Here's how the part is built. I have some questions about the finished solid (model axes, mm). A direction names the side the tool comes from. Give positions to 0.01 mm unless a question says otherwise; leave off trailing zeros. Write each loop counter-clockwise with the first axis right and the second up, starting at its lowest first coordinate (ties: lowest second). Pieces come first, ordered by that corner, then holes. Notation, with made-up numbers: (-26, 63) -> (-20, 63) arc R27 cw to (-20, 96) -> close; hole circle Ø10 at (18.25, 16.25). An arc over 180 degrees is marked (long way). Use CSV: the item, a comma, the result in double quotes. Start each with the question number.
(1) Suppose I cut it at C-C on y = 40. List the corners of the cut face in (x, z) for me, plus the area to 3 significant figures.
(2) Suppose I cut it at B-B on x = 21.4. List the corners of the cut face in (y, z) for me.
(3) If we mould it in two halves opening along X, with no side actions, what happens to faces 1 (the flat face through (0, 27, 0)), 2 (the cylindrical face through (-13.47, 54.64, 1.58)), 3 (the cylindrical face through (-32.287, 10.752, 1.578))? For each: pulls with the +X half, pulls with the -X half, needs draft (parallel to the pull), parting line crosses it, or undercut.
(4) For pin 1 Ø4.5 at (x, y) = (0, 17.5) entering from +Z; pin 2 Ø1.6 at (x, z) = (-18.5, 1.5) entering from +Y; pin 3 Ø1 at (y, z) = (30.5, 1.5) entering from -X; pin 4 Ø1 at (y, z) = (25.5, 1.5) entering from -X, each with a flat end and sliding along its axis, tell me the tip position at first contact or that it passes through.
(5) I need wall thicknesses on L1, parallel to Y at x = 0, z = 1.45; L2, parallel to Y at x = 21.4, z = 2.2; L3, parallel to Y at x = 2, z = 1.45. Which ranges of each line are inside material? Lowest first, please. Write a range as [from, to].
(6) Suppose I cut it at A-A on z = 1.45. Give the number of separate pieces and of enclosed holes in the cut face, plus the area to 3 significant figures.
(7) Suppose I cut it at D-D on y = 62.5. List the corners of the cut face in (x, z) for me.
(8) Which directions (+Z, -Z, +X, -X, +Y, -Y) give clear straight access to the entire face, cutting with the end or side of a thin tool? Please do faces 4 (the cylindrical face through (10.113, 40.15, 1.578)), 5 (the flat face through (-12.3, 42, 2)).
from build123d import *

# Parameters (mm, degrees)
SKETCH1_W                          = 19.6
SKETCH1_H                          = 44.5
SKETCH1_R                          = 2.5527
SKETCH1_R_2                        = 7
SKETCH1_H_2                        = 15
BOSS_EXTRUDE1_DEPTH                = 3.2
SKETCH2_W                          = 23.2
SKETCH2_H                          = 15
SKETCH2_R                          = 2.5527
T_SHAPE_EXTENSION_DEPTH            = 3.2
ASYMMETRIC_TRIANGLE_SUPPORTS_DEPTH = 3.2
FILLET1_R                          = 1.5
FILLET2_R                          = 2.5
FILLET3_R                          = 0.5
FILLET4_R                          = 2.5


with BuildPart() as part:
    # Sketch1 → Boss-Extrude1 (new body)
    # profile 1 of 2: a face of its own
    with BuildSketch(Plane.XY):
        with Locations((0, 47.25)):
            Rectangle(SKETCH1_W, SKETCH1_H)
        with Locations((0, 62.5)):
            Circle(SKETCH1_R, mode=Mode.SUBTRACT)
        with Locations((0, 40)):
            Circle(SKETCH1_R_2, mode=Mode.SUBTRACT)
    # profile 2 of 2: a face of its own
    with BuildSketch(Plane.XY):
        with Locations((0, 17.5)):
            Rectangle(SKETCH1_W, SKETCH1_H_2)
        with Locations((0, 17.5)):
            Circle(SKETCH1_R, mode=Mode.SUBTRACT)
    extrude(amount=BOSS_EXTRUDE1_DEPTH)

    # Sketch2 → T-shape Extension (add)
    # profile 1 of 2: a face of its own
    with BuildSketch(Plane.XY.offset(3.2)):
        with Locations((21.4, 17.5)):
            Rectangle(SKETCH2_W, SKETCH2_H)
        with Locations((21.4, 17.5)):
            Circle(SKETCH2_R, mode=Mode.SUBTRACT)
    # profile 2 of 2: a face of its own
    with BuildSketch(Plane.XY.offset(3.2)):
        with Locations((-21.4, 17.5)):
            Rectangle(SKETCH2_W, SKETCH2_H)
        with Locations((-21.4, 17.5)):
            Circle(SKETCH2_R, mode=Mode.SUBTRACT)
    extrude(amount=-T_SHAPE_EXTENSION_DEPTH)

    # Sketch8 → Asymmetric Triangle Supports (add)
    # profile 1 of 2: a face of its own
    with BuildSketch(Plane.XY.offset(3.2)):
        Polygon((-9.8, 69.5), (-33, 25), (-9.8, 25), align=None)
        Polygon((-12.3, 59.296922481), (-12.3, 27.5), (-28.877271945, 27.5), align=None, mode=Mode.SUBTRACT)
    # profile 2 of 2: a face of its own
    with BuildSketch(Plane.XY.offset(3.2)):
        Polygon((9.8, 25), (33, 25), (9.8, 40), align=None)
        Polygon((12.3, 27.5), (12.3, 35.40659498), (24.528866903, 27.5), align=None, mode=Mode.SUBTRACT)
    extrude(amount=-ASYMMETRIC_TRIANGLE_SUPPORTS_DEPTH)

    # Fillet1
    fillet1_edges = [part.edges().sort_by_distance(p)[0] for p in [
        (-28.877271945, 27.5, 1.6),
        (-12.3, 59.296922481, 1.6),
    ]]
    fillet(fillet1_edges, radius=FILLET1_R)

    # Fillet2
    fillet2_edges = [part.edges().sort_by_distance(p)[0] for p in [
        (-12.3, 27.5, 1.6),
    ]]
    fillet(fillet2_edges, radius=FILLET2_R)

    # Fillet3
    fillet3_edges = [part.edges().sort_by_distance(p)[0] for p in [
        (24.528866903, 27.5, 1.6),
        (12.3, 27.5, 1.6),
        (12.3, 35.40659498, 1.6),
    ]]
    fillet(fillet3_edges, radius=FILLET3_R)

    # Fillet4
    fillet4_edges = [part.edges().sort_by_distance(p)[0] for p in [
        (-9.8, 69.5, 1.6),
        (9.8, 69.5, 1.6),
        (33, 25, 1.6),
        (33, 10, 1.6),
        (-33, 10, 1.6),
        (-33, 25, 1.6),
        (9.8, 40, 1.6),
    ]]
    fillet(fillet4_edges, radius=FILLET4_R)


solid = part.part
Geometry says:
1,outline,"(-25.18, 0) -> (-22.36, 0) -> (-22.36, 3.2) -> (-25.18, 3.2) -> close; (-12.3, 0) -> (-7, 0) -> (-7, 3.2) -> (-12.3, 3.2) -> close; (7, 0) -> (10.2, 0) -> (10.2, 3.2) -> (7, 3.2) -> close"
1,area,"36.2 mm²"
2,outline,"(10, 0) -> (14.95, 0) -> (14.95, 3.2) -> (10, 3.2) -> close; (20.05, 0) -> (27.5, 0) -> (27.5, 3.2) -> (20.05, 3.2) -> close; (29.52, 0) -> (32.5, 0) -> (32.5, 3.2) -> (29.52, 3.2) -> close"
3,face 1,"needs draft"
3,face 2,"undercut"
3,face 3,"pulls with the -X half"
4,pin 1,"through"
4,pin 2,"y = 54.35"
4,pin 3,"x = -30.39"
4,pin 4,"x = -32.92"
5,L1,"[10, 14.95], [20.05, 33], [47, 59.95], [65.05, 69.5]"
5,L2,"[10, 14.95], [20.05, 27.5], [29.52, 32.5]"
5,L3,"[10, 15.91], [19.09, 33.29], [46.71, 60.91], [64.09, 69.5]"
6,separate pieces,"1"
6,enclosed holes,"7"
6,area,"2,010 mm²"
7,outline,"(-13.45, 0) -> (-2.55, 0) -> (-2.55, 3.2) -> (-13.45, 3.2) -> close; (2.55, 0) -> (9.8, 0) -> (9.8, 3.2) -> (2.55, 3.2) -> close"
8,face 4,"+Z, -Z, +X, +Y"
8,face 5,"+Z, -Z"
